Here's how the part is built. I have some questions about the finished solid (model axes, mm). A direction names the side the tool comes from. Coordinates: 2 decimals unless noted, no trailing zeros. Write each loop counter-clockwise with the first axis right and the second up, starting at its lowest first coordinate (ties: lowest second). Pieces come first, ordered by that corner, then holes. Notation, with made-up numbers: (37.5, 12) -> (64.5, 12) arc R15 cw to (64.5, 41) -> close; hole circle Ø9 at (6.25, 47.25). An arc over 180 degrees is marked (long way). Put each result on its own line as item: value. Start each with the question number.
Item 1: I want a section at D-D, the plane x = 88.5. List the corners of the cut face in (y, z) for me (3 decimals), then the cut area to 3 significant figures.
Item 2: I need wall thicknesses on line 1 (Y direction, x = 14, z = 16.5); line 2 (Z direction, x = -9.5, y = -24) (3 decimals); line 3 (Z direction, x = 88, y = 16.5) (3 decimals). Which ranges of each line are inside material? Lowest first, please. Write a range as [from, to].
Item 3: I want a section at A-A, the plane z = 2.5. List the corners of the cut face in (x, y) for me (3 decimals), then the cut area to 3 significant figures.
Item 4: I want a section at C-C, the plane x = 72.5. List the corners of the cut face in (y, z) for me (3 decimals).
Item 5: On a 3-axis mill with a long thin cutter (end or side, diameter ignored), from which of +Z, -Z, +X, -X, +Y, -Y can I reach the whole of each face in a straight line? I mean faces 1 (the face through (86, 0, 38.1)), 2 (the face through (60, 0, 61.925)), 3 (the face through (22.225, -17, 18)), 4 (the face through (-3, 7.938, 30)). Say none if no direction works.
Item 6: I want a section at B-B, the plane y = 44.5. List the corners of the cut face in (x, z) for me (3 decimals), then the cut area to 3 significant figures.
Item 7: For pin 1 (8 mm diameter, centred on x = 69.5, z = 34, fed in from -Y); pin 2 (4 mm diameter, centred on y = 5, z = 34.5, fed in from -X); pin 3 (8 mm diameter, centred on x = 30.5, y = 43, fed in from +Z) (3 decimals); pin 4 (5 mm diameter, centred on y = 15.5, z = 20.5, fed in from -X) (3 decimals), each with a flat end and sliding along its axis, tell me the tip position at first contact or that it passes through.
Item 8: If we mould it in two halves opening along X, with no side actions, what happens to faces 5 (the face through (1, 35, 9.525)), 6 (the face through (32.137, -16.791, 51.374)), 7 (the face through (58, 0, 42.875)), 8 (the face through (45.8, -0.4, 38.1))? For each: released by +X, released by -X, zero draft, split by the parting line, or undercut.
from build123d import *

# Parameters (mm, degrees)
F1_DEPTH = 63.5
F0_W     = 19.9390054388
F0_H     = 19.0500000358
F2_DEPTH = 25.4
F3_DEPTH = 7.9375
F0_W_2   = 25.4
F0_H_2   = 28.575
F5_R     = 5.08


with BuildPart() as f1:
    # F0 (on Front) → F1 (new body, symmetric)
    with BuildSketch(Plane.XZ):
        Polygon((22.2249999642, 9.525), (-41.275, 9.525), (-41.275, -9.525), (41.275, -9.525), (41.275, 9.525), align=None)
    extrude(amount=F1_DEPTH, both=True)

    # F0 (on Front) → F2 (join, symmetric)
    with BuildSketch(Plane.XZ):
        with BuildLine():
            Line((22.2249999642, 27.0002), (22.2249999642, 9.525))
            Line((22.2249999642, 9.525), (41.275, 9.525))
            Line((41.275, 9.525), (41.275, 27.0002))
            ThreePointArc((41.275, 27.0002), (45.9246798487, 38.2255201513), (57.15, 42.8752))
            Line((57.15, 42.8752), (60.325, 42.8752))
            Line((60.325, 42.8752), (60.325, 61.9252000358))
            Line((60.325, 61.9252000358), (57.15, 61.9252000358))
            add(Edge.make_bspline(
                [(55.5009997986, 61.8862491577), (56.0491292612, 61.9014539237), (56.5988031448, 61.9144444348), (57.15, 61.9252000358)],
                knots=[110.4291039898, 110.4291039898, 110.4291039898, 110.4291039898, 111.5045361803, 111.5045361803, 111.5045361803, 111.5045361803], degree=3))
            ThreePointArc((55.5009997986, 61.8862491577), (31.8780099756, 51.1058455566), (22.2249999642, 27.0002))
        make_face()
        with Locations((70.2945027194, 52.4002000179)):
            Rectangle(F0_W, F0_H)
    extrude(amount=F2_DEPTH, both=True)

    # F0 (on Front) → F3 (join, symmetric)
    with BuildSketch(Plane.XZ):
        with BuildLine():
            add(Edge.make_bspline(
                [(-41.275, 9.525), (-40.7824539229, 35.4168247644), (-0.7828328366, 60.3249711005), (55.5009997986, 61.8862491577)],
                knots=[0, 0, 0, 0, 110.4291039898, 110.4291039898, 110.4291039898, 110.4291039898], degree=3))
            Line((-41.275, 9.525), (22.2249999642, 9.525))
            Line((22.2249999642, 9.525), (22.2249999642, 27.0002))
            ThreePointArc((22.2249999642, 27.0002), (31.8780099756, 51.1058455566), (55.5009997986, 61.8862491577))
        make_face()
    extrude(amount=F3_DEPTH, both=True)

    # F0 (on Front) → F4 (revolve)
    with BuildSketch(Plane.XZ):
        with Locations((98.425, 52.3875)):
            Rectangle(F0_W_2, F0_H_2)
    revolve(axis=Axis((85.725, 0, 52.3875), (0, 0, 1)))

    # F5
    f5_edges = [f1.edges().sort_by_distance(p)[0] for p in [
        (-41.275, -63.5, 0),
        (41.275, -63.5, 0),
        (41.275, 63.5, 0),
        (-41.275, 63.5, 0),
    ]]
    fillet(f5_edges, radius=F5_R)


solid = f1.part
Calculated:
1. outline: (-25.248, 38.1) -> (25.248, 38.1) -> (25.248, 66.675) -> (-25.248, 66.675) -> close
1. area: 1,440 mm2
2. line 1: y = [-7.94, 7.94]
2. line 2: z = [-9.525, 9.525]
2. line 3: z = [38.1, 66.675]
3. outline: (-41.275, -58.42) arc R5.08 ccw to (-36.195, -63.5) -> (36.195, -63.5) arc R5.08 ccw to (41.275, -58.42) -> (41.275, 58.42) arc R5.08 ccw to (36.195, 63.5) -> (-36.195, 63.5) arc R5.08 ccw to (-41.275, 58.42) -> close
3. area: 10,500 mm2
4. outline: (-25.4, 42.875) -> (-21.685, 42.875) -> (-21.685, 38.1) -> (21.685, 38.1) -> (21.685, 42.875) -> (25.4, 42.875) -> (25.4, 61.925) -> (21.685, 61.925) -> (21.685, 66.675) -> (-21.685, 66.675) -> (-21.685, 61.925) -> (-25.4, 61.925) -> close
5. face 1: -Z, +X, +Y, -Y
5. face 2: +Z, -X
5. face 3: +Z, -X, -Y
5. face 4: +Z, -X, +Y
6. outline: (-41.275, -9.525) -> (41.275, -9.525) -> (41.275, 9.525) -> (-41.275, 9.525) -> close
6. area: 1,570 mm2
7. pin 1: passes through
7. pin 2: stops at x = -30.27
7. pin 3: stops at z = 9.525
7. pin 4: stops at x = 22.225
8. face 5: zero draft
8. face 6: released by -X
8. face 7: undercut
8. face 8: undercut
